from build123d import *

# Parameters (mm, degrees)
CHAMFER1_SIZE               = 8.89
F_19_0_166_DIAMETER_HOLE1_D = 4.2164


with BuildPart() as part:
    # Sketch1 → Revolve1 (revolve)
    with BuildSketch(Plane.XY, mode=Mode.PRIVATE) as revolve1_sk:
        Polygon((-29.337, 0), (-41.275, 0), (-41.275, -9.525), (0, -9.525), (0, 0), (-21.1455, 0), (-21.1455, 9.525), (-29.337, 9.525), align=None)
    revolve(revolve1_sk.sketch.rotate(Axis((0, -9.525, 0), (0, 1, 0)), 270), axis=Axis((0, -9.525, 0), (0, 1, 0)))

    # Chamfer1
    chamfer1_edges = [part.edges().sort_by_distance(p)[0] for p in [
        (0, -9.525, 41.275),
    ]]
    chamfer(chamfer1_edges, length=CHAMFER1_SIZE)

    # #19 (0.166) Diameter Hole1 (through all)
    with Locations(Plane(origin=(0, -9.525, 0), x_dir=(0, 0, -1), z_dir=(0, -1, 0))):
        with Locations((0, 0)):
            Hole(F_19_0_166_DIAMETER_HOLE1_D / 2)


solid = part.part
For this review, take the finished solid that the model builds, in its own axes (mm). A direction names the side the tool comes from. Round coordinates to 2 decimals unless told otherwise and drop trailing zeros. Order: outer loops, then holes, each group sorted by start corner. A loop starts at its lowest first (then second) coordinate and runs counter-clockwise, first axis right, second up. Notation, with made-up numbers: M 83.25,15 L 90.25,15 A27 cw 90.25,41 Z; hole C 16.25,-2 d7. An arc over 180 degrees is marked long. Use a Markdown table: item, result. Add a question column.
Item 1: Add section A-A, the plane z = 0. Give the boundary of the cut face in (x, y) (1 decimal), then the cut area to 3 significant figures.
Item 2: Add section B-B, the plane x = 0. Give the boundary of the cut face in (y, z) (1 decimal), then the cut area to 3 significant figures.
Item 3: Add section C-C, the plane y = 4.75. Give the boundary of the cut face in (x, z).
Item 4: Mouldability with a two-part tool opening along X and no side actions: class faces 3 (the flat face through (7, -9.525, 0)), 4 (the cylindrical face through (-14.291, 4.829, 15.585)), 5 (the cylindrical face through (-29.087, 4.696, 3.819)) as released by +X, released by -X, zero draft, split by the parting line, or undercut.
Item 5: Tool access review of faces 1 (the conical face through (-32.54, -9.09, 4.27)), 2 (the flat face through (4, 0, 0)): name each direction out of +Z, -Z, +X, -X, +Y, -Y from which nothing blocks a thin tool from reaching the whole face with its end or side.
Item 6: Insertion check: pin 1 (8 mm diameter, centred on y = -5, z = -6, fed in from -X); pin 2 (2 mm diameter, centred on x = -20, y = -5, fed in from -Z); pin 3 (6 mm diameter, centred on x = 25.5, z = -28, fed in from +Y). Each pin has a flat end and moves straight along its axis. Give the tip position at first contact, or say it passes through.
Item 7: To check wall thickness, follow line 1 along X through (y, z) = (4.5, 0); line 2 along Y through (x, z) = (4.5, 2) (3 decimals); line 3 along X through (y, z) = (-1.75, 0). State the ranges of each line that lie inside material, in increasing order.
Geometry results:
| question | item | result |
|---|---|---|
| 1 | outline | M -41.3,-0.6 L -32.4,-9.5 L -2.1,-9.5 L -2.1,0 L -21.1,0 L -21.1,9.5 L -29.3,9.5 L -29.3,0 L -41.3,0 Z; M 2.1,-9.5 L 32.4,-9.5 L 41.3,-0.6 L 41.3,0 L 29.3,0 L 29.3,9.5 L 21.1,9.5 L 21.1,0 L 2.1,0 Z |
| 1 | area | 823 mm² |
| 2 | outline | M -9.5,-32.4 L -0.6,-41.3 L 0,-41.3 L 0,-29.3 L 9.5,-29.3 L 9.5,-21.1 L 0,-21.1 L 0,-2.1 L -9.5,-2.1 Z; M -9.5,2.1 L 0,2.1 L 0,21.1 L 9.5,21.1 L 9.5,29.3 L 0,29.3 L 0,41.3 L -0.6,41.3 L -9.5,32.4 Z |
| 2 | area | 823 mm² |
| 3 | outline | C 0,0 d58.67; hole C 0,0 d42.29 |
| 4 | face 3 | zero draft |
| 4 | face 4 | undercut |
| 4 | face 5 | split by the parting line |
| 5 | face 1 | -Y |
| 5 | face 2 | +Y |
| 6 | pin 1 | stops at x = -40.51 |
| 6 | pin 2 | stops at z = -32.36 |
| 6 | pin 3 | stops at y = 0 |
| 7 | line 1 | x = -29.34 to -21.15, 21.15 to 29.34 |
| 7 | line 2 | y = -9.525 to 0 |
| 7 | line 3 | x = -40.16 to -2.11, 2.11 to 40.16 |
